For this review, take the finished solid that the model builds, in its own axes (mm). A direction names the side the tool comes from. Give positions to 0.01 mm unless a question says otherwise; leave off trailing zeros. Loops run counter-clockwise (first coordinate to the right, second up) from the corner with the lowest first, then second, coordinate; pieces in that order, holes last. Notation, with made-up numbers: (77, 34.5) - (101, 34.5) arc R18 ccw to (101, 67.5) - close; hole circle Ø3 at (24.25, 16.5). An arc over 180 degrees is marked (long way). Put each result on its own line as item: value. Start each with the question number.
from build123d import *

# Parameters (mm, degrees)
F1_DEPTH = 50.8
F3_DEPTH = 101.601
F6_T     = -9.525


with BuildPart() as f1:
    # F0 (on Front) → F1 (new body)
    with BuildSketch(Plane.XZ):
        Polygon((0, 88.9), (0, 0), (85.924531, 0), (101.6, 88.9), align=None)
    extrude(amount=F1_DEPTH)

    # F2 (on Right) → F3 (cut, through all)
    with BuildSketch(Plane.YZ):
        Polygon((-35.124531, 0), (-50.8, 88.9), (-50.8, 0), align=None)
    extrude(amount=F3_DEPTH, mode=Mode.SUBTRACT)

    # F4: F1 across plane


with BuildPart() as f1_1:
    add(f1.part)
    add(f1.part.mirror(Plane.XZ))

    # F5: F1 across plane


with BuildPart() as f1_2:
    add(f1_1.part)
    add(f1_1.part.mirror(Plane.YZ))

    # F6
    f6_openings = [f1_2.faces().sort_by_distance(p)[0] for p in [
        (0, 0, 88.9),
    ]]
    offset(amount=F6_T, openings=f6_openings)


solid = f1_2.part
1) Take a section at A-A on y = -7. State the section outline as (x, z) points (3 decimals), and give its area (3 significant figures).
2) Mouldability with a two-part tool opening along Y and no side actions: class faces 3 (the flat face through (-84.832, -0.576, 48.657)), 4 (the flat face through (0, -42, 88.9)), 5 (the flat face through (1.422, 42.853, 43.828)) as released by +Y, released by -Y, zero draft, split by the parting line, or undercut.
3) Take a section at C-C on x = -22.5. State the section outline as (y, z) points (3 decimals), and give its area (3 significant figures).
4) Insertion check: P1, Ø1, axis at x = -30.5, z = 75, coming from the -Y side; P2, Ø1.5, axis at x = 56.5, z = 56, coming from the -Y side; P3, Ø4, axis at y = -32, z = 21, coming from the +X side; P4, Ø12, axis at x = 7, y = 9, coming from the -Z side. Each pin has a flat end and moves straight along its axis. Give the tip position at first contact, or say it passes through.
5) Take a section at B-B on z = 59.5. State the section outline as (x, y) points.
6) Machinability: for faces 1 (the flat face through (1.422, -42.853, 43.828)), 2 (the flat face through (84.832, -0.576, 48.657)), which of the approach directions +Z, -Z, +X, -X, +Y, -Y give a long, thin tool a straight path to every point of the face, cutting with its end or side? Answer none if there is none.
7) Take a section at D-D on z = 76. State the section outline as (x, y) points, and give its area (3 significant figures).
8) Wall thickness on probe 1 along Z at (x, y) = (68.5, 22.5) (3 decimals); probe 2 along X at (y, z) = (0, 59.5); probe 3 along Y at (x, z) = (-81.5, 61): over which ranges is each line inside the solid? List them lowest first.
Answers follow:
1. outline: (-101.6, 88.9) - (-85.925, 0) - (85.925, 0) - (101.6, 88.9) - (91.928, 88.9) - (77.932, 9.525) - (-77.932, 9.525) - (-91.928, 88.9) - close
1. area: 3,190 mm2
2. face 3: undercut
2. face 4: zero draft
2. face 5: released by +Y
3. outline: (-50.8, 88.9) - (-35.125, 0) - (35.125, 0) - (50.8, 88.9) - (41.128, 88.9) - (27.132, 9.525) - (-27.132, 9.525) - (-41.128, 88.9) - close
3. area: 2,220 mm2
4. P1: y = -48.44
4. P2: y = -45.13
4. P3: x = 89.98
4. P4: z = 0
5. outline: (-96.42, -45.62) - (96.42, -45.62) - (96.42, 45.62) - (-96.42, 45.62) - close; hole (-86.74, -35.94) - (86.74, -35.94) - (86.74, 35.94) - (-86.74, 35.94) - close
6. face 1: -Z, +X, -X, -Y
6. face 2: +Z
7. outline: (-99.33, -48.53) - (99.33, -48.53) - (99.33, 48.53) - (-99.33, 48.53) - close; hole (-89.65, -38.85) - (89.65, -38.85) - (89.65, 38.85) - (-89.65, 38.85) - close
7. area: 5,350 mm2
8. probe 1: 0 to 9.525
8. probe 2: -96.42 to -86.74, 86.74 to 96.42
8. probe 3: -45.88 to -36.21, 36.21 to 45.88
